from build123d import *

# Parameters (mm, degrees)
SKETCH1_R           = 6
BOSS_EXTRUDE1_DEPTH = 4
SKETCH2_R           = 4
BOSS_EXTRUDE2_DEPTH = 29
SKETCH3_R           = 2.5
BOSS_EXTRUDE3_DEPTH = 7
CHAMFER1_SIZE       = 0.5
CHAMFER2_SIZE       = 1
SKETCH4_R           = 2.5
CUT_EXTRUDE1_DEPTH  = 1
FILLET1_R           = 0.5


with BuildPart() as part:
    # Sketch1 → Boss-Extrude1 (new body)
    with BuildSketch(Plane(origin=(0, 0, 0), x_dir=(0, 0, -1), z_dir=(1, 0, 0))):
        Circle(SKETCH1_R)
    extrude(amount=BOSS_EXTRUDE1_DEPTH)

    # Sketch2 → Boss-Extrude2 (add)
    with BuildSketch(Plane(origin=(4, 0, 0), x_dir=(0, 0, -1), z_dir=(1, 0, 0))):
        Circle(SKETCH2_R)
    extrude(amount=BOSS_EXTRUDE2_DEPTH)

    # Sketch3 → Boss-Extrude3 (add)
    with BuildSketch(Plane(origin=(33, 0, 0), x_dir=(0, 0, -1), z_dir=(1, 0, 0))):
        Circle(SKETCH3_R)
    extrude(amount=BOSS_EXTRUDE3_DEPTH)

    # Chamfer1
    chamfer1_edges = [part.edges().sort_by_distance(p)[0] for p in [
        (40, 0, 2.5),
    ]]
    chamfer(chamfer1_edges, length=CHAMFER1_SIZE)

    # Chamfer2
    chamfer2_edges = [part.edges().sort_by_distance(p)[0] for p in [
        (0, 0, 6),
    ]]
    chamfer(chamfer2_edges, length=CHAMFER2_SIZE)

    # Sketch4 → Cut-Extrude1 (cut)
    with BuildSketch(Plane.ZY):
        Circle(SKETCH4_R)
    extrude(amount=-CUT_EXTRUDE1_DEPTH, mode=Mode.SUBTRACT)

    # Fillet1
    fillet1_edges = [part.edges().sort_by_distance(p)[0] for p in [
        (0, 0, -2.5),
    ]]
    fillet(fillet1_edges, radius=FILLET1_R)


solid = part.part
Design review of the part built by this model. Coordinates are the model's own, in mm. A direction names the side the tool comes from. Coordinates: 2 decimals unless noted, no trailing zeros. Order: outer loops, then holes, each group sorted by start corner. A loop starts at its lowest first (then second) coordinate and runs counter-clockwise, first axis right, second up.
Item 1: For line 1 (X direction, y = 4.5, z = -1.25); line 2 (X direction, y = 0, z = -0.5); line 3 (Z direction, x = 32.5, y = -0.25), list the stretches that pass through material, from the lowest coordinate up.
Item 2: Take a section at C-C, the plane x = 27.5. Write out the cut boundary in (y, z), then the cut area to 3 significant figures.
Item 3: For pin 1 Ø6 at (x, z) = (22, 4.5) entering from +Y; pin 2 Ø4 at (x, z) = (26.5, 3) entering from +Y; pin 3 Ø1.5 at (y, z) = (0.5, 0.5) entering from -X, all flat-tipped, find the tip position at first contact; note any pin that passes through.
Item 4: Take a section at A-A, the plane z = 0. Write out the cut boundary in (x, y), then the cut area to 3 significant figures.
Item 5: For faces 4 (the cylindrical face through (0.75, -2.44, -0.54)), 5 (the flat face through (40, 0, 0)), 6 (the flat face through (33, 2, -2)), list the 3-axis set-ups (+Z, -Z, +X, -X, +Y, -Y) from which the entire face can be reached by the end or side of a thin tool; tool diameter is ignored.
Item 6: The part is to be moulded in two halves that separate along Y. For faces 1 (the flat face through (0, -3.3, 0.1)), 2 (the cylindrical face through (2, 0, 6)), 3 (the flat face through (1, 0, 0)), say which applies: pulls with the +Y half, pulls with the -Y half, needs draft (parallel to the pull), parting line crosses it, or undercut.
The answers:
1. line 1: x = 0 to 4
1. line 2: x = 1 to 40
1. line 3: z = -3.99 to 3.99
2. outline: circle Ø8 at (0, 0)
2. area: 50.3 mm2
3. pin 1: stops at y = 3.71
3. pin 2: stops at y = 3.87
3. pin 3: stops at x = 1
4. outline: (0, -5) - (1, -6) - (4, -6) - (4, -4) - (33, -4) - (33, -2.5) - (39.5, -2.5) - (40, -2) - (40, 2) - (39.5, 2.5) - (33, 2.5) - (33, 4) - (4, 4) - (4, 6) - (1, 6) - (0, 5) - (0, 3) arc R0.5 ccw to (0.5, 2.5) - (1, 2.5) - (1, -2.5) - (0.5, -2.5) arc R0.5 ccw to (0, -3) - close
4. area: 309 mm2
5. face 4: -X
5. face 5: +Z, -Z, +X, +Y, -Y
5. face 6: +X
6. face 1: needs draft
6. face 2: parting line crosses it
6. face 3: undercut
